from build123d import *

# Parameters (mm, degrees)
SKETCH_2_W           = 43
SKETCH_2_H           = 10
SKETCH_2_W_2         = 10
SKETCH_2_H_2         = 15
EXTRUDE_1_DEPTH      = 1
EXTRUDE_2_DEPTH      = 4
EXTRUDE_2_DEPTH_BACK = 1
SKETCH_4_W           = 15
SKETCH_4_H           = 10
SKETCH_4_W_2         = 10
SKETCH_4_H_2         = 15
EXTRUDE_3_DEPTH      = 2


with BuildPart() as part:
    # 草图2 → 凸台-拉伸1 (new body)
    with BuildSketch(Plane(origin=(0, 0, 0), x_dir=(1, 0, 0), z_dir=(0, 1, 0))):
        with Locations((-7.5, 0)):
            Rectangle(SKETCH_2_W, SKETCH_2_H)
        with Locations((9, 12.5)):
            Rectangle(SKETCH_2_W_2, SKETCH_2_H_2)
        with Locations((9, -12.5)):
            Rectangle(SKETCH_2_W_2, SKETCH_2_H_2)
    extrude(amount=EXTRUDE_1_DEPTH)

    # 草图3 → 凸台-拉伸2 (add, two sides)
    with BuildSketch(Plane(origin=(0, 1, 0), x_dir=(1, 0, 0), z_dir=(0, 1, 0))) as extrude_2_sk:
        Polygon((15, -21), (15, 21), (3, 21), (3, 6), (-30, 6), (-30, -6), (3, -6), (3, -21), align=None)
        Polygon((14, -20), (14, 20), (4, 20), (4, 5), (-29, 5), (-29, -5), (4, -5), (4, -20), align=None, mode=Mode.SUBTRACT)
    extrude(amount=EXTRUDE_2_DEPTH)
    extrude(extrude_2_sk.sketch, amount=-EXTRUDE_2_DEPTH_BACK)

    # 草图4 → 凸台-拉伸3 (add)
    with BuildSketch(Plane(origin=(0, 1, 0), x_dir=(1, 0, 0), z_dir=(0, 1, 0))):
        with Locations((-21.5, 0)):
            Rectangle(SKETCH_4_W, SKETCH_4_H)
        with Locations((9, 12.5)):
            Rectangle(SKETCH_4_W_2, SKETCH_4_H_2)
        with Locations((9, -12.5)):
            Rectangle(SKETCH_4_W_2, SKETCH_4_H_2)
    extrude(amount=EXTRUDE_3_DEPTH)


solid = part.part
Read the model definition and answer for the solid it produces. Units are mm, in the model's axes. A direction names the side the tool comes from. Round coordinates to 2 decimals unless told otherwise and drop trailing zeros. Write each loop counter-clockwise with the first axis right and the second up, starting at its lowest first coordinate (ties: lowest second). Pieces come first, ordered by that corner, then holes. Notation, with made-up numbers: M 25,62.25 L 81,62.25 A21 cw 81,99.25 Z; hole C 64,26 d7. An arc over 180 degrees is marked long. Use a Markdown table: item, result.
1) The part is cut by section C-C (x = -23). Write down the section's boundary in (y, z).
Answers follow:
| item | result |
|---|---|
| outline | M 0,-6 L 5,-6 L 5,-5 L 3,-5 L 3,5 L 5,5 L 5,6 L 0,6 Z |
2) A tool of negligible diameter and unlimited length cuts with its end or side. For faces 4 (the flat face through (3, 3, 13)), 5 (the flat face through (-22, 3, 0)), 6 (the flat face through (-13, 3, -6)), from which of +Z, -Z, +X, -X, +Y, -Y can it reach the whole face along a straight path? Write none if from no direction.
Answers follow:
| item | result |
|---|---|
| face 4 | +Z, -X, +Y, -Y |
| face 5 | +Y |
| face 6 | -Z, -X, +Y, -Y |
3) For a pull along Z with two mould halves and no side action, classify faces 1 (the flat face through (-30, 3, 0)), 2 (the flat face through (-29, 4, 0)), 3 (the flat face through (9, 3, -21)) as pulls with the +Z half, pulls with the -Z half, needs draft (parallel to the pull), parting line crosses it, or undercut.
Answers follow:
| item | result |
|---|---|
| face 1 | needs draft |
| face 2 | undercut |
| face 3 | pulls with the -Z half |
4) Straight lines are drawn through the part: line 1 along X through (y, z) = (3.6, 11); line 2 along Z through (x, y) = (2, 1.35); line 3 along Z through (x, y) = (7.5, 4.25). For each, find the intervals that lie inside material, in ascending order. Write a range as [from, to].
Answers follow:
| item | result |
|---|---|
| line 1 | x = [3, 4], [14, 15] |
| line 2 | z = [-6, -5], [5, 6] |
| line 3 | z = [-21, -20], [20, 21] |
5) Flat-ended cylindrical pins translate along their axes: pin 1 (3 mm diameter, centred on x = -1, z = -0.5, fed in from +Y); pin 2 (12 mm diameter, centred on x = -4, z = -4, fed in from +Y); pin 3 (2 mm diameter, centred on y = 3.5, z = 10, fed in from -X); pin 4 (3 mm diameter, centred on x = 7.5, z = 12, fed in from +Y). Find the tip coordinate at first contact, or state that the pin passes through.
Answers follow:
| item | result |
|---|---|
| pin 1 | stops at y = 1 |
| pin 2 | stops at y = 5 |
| pin 3 | stops at x = 3 |
| pin 4 | stops at y = 3 |
6) The part is cut by section B-B (z = -16). Write down the section's boundary in (x, y).
Answers follow:
| item | result |
|---|---|
| outline | M 3,0 L 15,0 L 15,5 L 14,5 L 14,3 L 4,3 L 4,5 L 3,5 Z |
7) The part is cut by section D-D (x = 7.5). Write down the section's boundary in (y, z), plus the area to 3 significant figures.
Answers follow:
| item | result |
|---|---|
| outline | M 0,-21 L 5,-21 L 5,-20 L 3,-20 L 3,-5 L 1,-5 L 1,5 L 3,5 L 3,20 L 5,20 L 5,21 L 0,21 Z |
| area | 110 mm2 |
8) The part is cut by section A-A (y = 4.5). Write down the section's boundary in (x, z).
Answers follow:
| item | result |
|---|---|
| outline | M -30,-6 L 3,-6 L 3,-21 L 15,-21 L 15,21 L 3,21 L 3,6 L -30,6 Z; hole M -29,-5 L 4,-5 L 4,-20 L 14,-20 L 14,20 L 4,20 L 4,5 L -29,5 Z |
